from build123d import *

# Parameters (mm, degrees)
AUFSATZ_LINEAR_AUSTRAGEN1_DEPTH = 50


with BuildPart() as part:
    # Skizze1 → Aufsatz-Linear austragen1 (new body)
    with BuildSketch(Plane.XY):
        Polygon((200, -9.5), (0, -9.5), (0, 0), (5, 1), (5, 0), (10, 1), (10, 0), (15, 1), (15, 0), (20, 1), (20, 0), (25, 1), (25, 0), (30, 1), (30, 0), (35, 1), (35, 0), (40, 1), (40, 0), (45, 1), (45, 0), (50, 1), (50, 0), (55, 1), (55, 0), (60, 1), (60, 0), (65, 1), (65, 0), (70, 1), (70, 0), (75, 1), (75, 0), (80, 1), (80, 0), (85, 1), (85, 0), (90, 1), (90, 0), (95, 1), (95, 0), (100, 1), (100, 0), (105, 1), (105, 0), (110, 1), (110, 0), (115, 1), (115, 0), (120, 1), (120, 0), (125, 1), (125, 0), (130, 1), (130, 0), (135, 1), (135, 0), (140, 1), (140, 0), (145, 1), (145, 0), (150, 1), (150, 0), (155, 1), (155, 0), (160, 1), (160, 0), (165, 1), (165, 0), (170, 1), (170, 0), (175, 1), (175, 0), (180, 1), (180, 0), (185, 1), (185, 0), (190, 1), (190, 0), (195, 1), (195, 0), (200, 1), (200, 0), align=None)
    extrude(amount=AUFSATZ_LINEAR_AUSTRAGEN1_DEPTH)


solid = part.part
Input: part model. Units: mm. Frame: model coordinates. A direction names the side the tool comes from. Give positions to 0.01 mm unless a question says otherwise; leave off trailing zeros. Order: outer loops, then holes, each group sorted by start corner. A loop starts at its lowest first (then second) coordinate and runs counter-clockwise, first axis right, second up.
Q1. Section A-A on x = 157. Output: boundary loops of the cut face in (y, z).
Checked values:
outline: (-9.5, 0) - (0.4, 0) - (0.4, 50) - (-9.5, 50) - close
Q2. Ray query, probe 1 along Y at (x, z) = (10.5, 14); probe 2 along Y at (x, z) = (128.5, 31). Return the intervals inside material, ascending.
Checked values:
probe 1: y = -9.5 to 0.1
probe 2: y = -9.5 to 0.7
Q3. Contact query for flat-ended pins moving along their axis: pin 1 Ø3 at (x, z) = (152, 28) entering from +Y; pin 2 Ø10 at (x, z) = (49.5, 31.5) entering from +Y. Output: stop coordinate, or through.
Checked values:
pin 1: stops at y = 0.7
pin 2: stops at y = 1
Q4. Section B-B on x = 188. Output: boundary loops of the cut face in (y, z).
Checked values:
outline: (-9.5, 0) - (0.6, 0) - (0.6, 50) - (-9.5, 50) - close
Q5. Set-up query: faces 1 (the flat face through (101, -4, 0)), 2 (the flat face through (72.5, 0.5, 24.6)). Return all of +Z, -Z, +X, -X, +Y, -Y with unobstructed straight access to the full face (end or side cutting, diameter ignored); none if empty.
Checked values:
face 1: -Z, +X, -X, +Y, -Y
face 2: +Z, -Z, +Y
